Verification items for the finished model (mm, model axes). A direction names the side the tool comes from. Round coordinates to 2 decimals unless told otherwise and drop trailing zeros. Write each loop counter-clockwise with the first axis right and the second up, starting at its lowest first coordinate (ties: lowest second). Pieces come first, ordered by that corner, then holes. Notation, with made-up numbers: (-5.5, 40.25) -> (4.5, 40.25) arc R29 cw to (4.5, 70.25) -> close; hole circle Ø6 at (54, 4.25). An arc over 180 degrees is marked (long way). Answer as a JSON object with one key per item and string values. Group by question number.
(1) Scan lines: L1, parallel to Y at x = 12.5, z = 0.6; L2, parallel to Z at x = -0.75, y = -2.5; L3, parallel to Y at x = 4, z = 6. Record each from-to range of solid material in increasing order. Write a range as from..to.
(2) Draft check along Y on faces 1 (the face through (13.31, 19.25, 0.76)), 2 (the face through (-14, -7, 1)), 3 (the face through (-0.71, 16.5, 14.96)), 4 (the face through (-9, 11, 5)). Enter one of: released by +Y, released by -Y, zero draft, split by the parting line, or undercut.
(3) Set-up check for faces 5 (the face through (0, -10, 2)), 6 (the face through (-1, 15, 11.5)), 7 (the face through (0, 16.117, 5)), 8 (the face through (9, 11, 5)): record each of +Z, -Z, +X, -X, +Y, -Y from which the full face is reachable in a straight line by a thin tool's end or side.
(4) Sectioned sample at B-B on y = -6. Record the cut outline in (x, z).
(5) Sectioned sample at A-A on x = 12.5. Record the cut outline in (y, z), and give its area (3 significant figures).
(6) Sectioned sample at D-D on y = 10. Record the cut outline in (x, z).
(7) Gauge pin test, flat ends, axial feed: pin 1 Ø2.5 at (x, z) = (0.5, 5.5) entering from +Y; pin 2 Ø0.6 at (y, z) = (-10.5, 2) entering from -X; pin 3 Ø6 at (x, z) = (7, 10) entering from -Y; pin 4 Ø5.5 at (x, y) = (-1, 9) entering from -Z. Record the tip position at first contact, or that the pin passes through.
(8) Sectioned sample at C-C on z = 5.75. Record the cut outline in (x, y), and give its area (3 significant figures).
```python
from build123d import *

# Parameters (mm, degrees)
SKETCH_1_W          = 30
SKETCH_1_H          = 40
EXTRUDE_1_DEPTH     = 1.5
SKETCH_2_R          = 1.5
CUT_EXTRUDE_1_DEPTH = 2.5
SKETCH_3_W          = 18
SKETCH_3_H          = 10
EXTRUDE_2_DEPTH     = 8
SKETCH_4_R          = 5
EXTRUDE_3_DEPTH     = 2
SKETCH_5_R          = 3.78256648
EXTRUDE_4_DEPTH     = 1
SKETCH_6_R          = 5.431564172
EXTRUDE_5_DEPTH     = 5
SKETCH_7_W          = 12
SKETCH_7_H          = 12
EXTRUDE_6_DEPTH     = 0.5


with BuildPart() as part:
    # 草图1 → 凸台-拉伸1 (new body)
    with BuildSketch(Plane.XY):
        Rectangle(SKETCH_1_W, SKETCH_1_H)
    extrude(amount=EXTRUDE_1_DEPTH)

    # 草图2 → 切除-拉伸1 (cut, through all)
    with BuildSketch(Plane.XY.offset(1.5)):
        with Locations((-12.5, 17.989454292)):
            Circle(SKETCH_2_R)
        with Locations((12.5, 17.989454292)):
            Circle(SKETCH_2_R)
        with Locations((-12.5, -7.010545708)):
            Circle(SKETCH_2_R)
        with Locations((12.5, -7.010545708)):
            Circle(SKETCH_2_R)
    extrude(amount=-CUT_EXTRUDE_1_DEPTH, mode=Mode.SUBTRACT)

    # 草图3 → 凸台-拉伸2 (add)
    with BuildSketch(Plane.XY.offset(1.5)):
        with Locations((0, 11.11683457)):
            Rectangle(SKETCH_3_W, SKETCH_3_H)
    extrude(amount=EXTRUDE_2_DEPTH)

    # 草图4 → 凸台-拉伸3 (add)
    with BuildSketch(Plane.XY.offset(9.5)):
        with Locations((0, 11.11683457)):
            Circle(SKETCH_4_R)
    extrude(amount=EXTRUDE_3_DEPTH)

    # 草图5 → 凸台-拉伸4 (add)
    with BuildSketch(Plane.XY.offset(11.5)):
        with Locations((0, 11.11683457)):
            Circle(SKETCH_5_R)
    extrude(amount=EXTRUDE_4_DEPTH)

    # 草图6 → 凸台-拉伸5 (add)
    with BuildSketch(Plane.XY.offset(12.5)):
        with Locations((0, 11.11683457)):
            Circle(SKETCH_6_R)
    extrude(amount=EXTRUDE_5_DEPTH)

    # 草图7 → 凸台-拉伸6 (add)
    with BuildSketch(Plane.XY.offset(1.5)):
        with Locations((0, -9.903085883)):
            Rectangle(SKETCH_7_W, SKETCH_7_H)
    extrude(amount=EXTRUDE_6_DEPTH)


solid = part.part
```
Computed values:
{
 "1": {"L1": "-20..-8.51, -5.51..16.49, 19.49..20", "L2": "0..1.5", "L3": "6.12..16.12"},
 "2": {"face 1": "undercut", "face 2": "undercut", "face 3": "split by the parting line", "face 4": "zero draft"},
 "3": {"face 5": "+Z, +X, -X, -Y", "face 6": "none", "face 7": "+X, -X, +Y", "face 8": "+Z, +X, +Y, -Y"},
 "4": {"outline": "(-15, 0) -> (-13.61, 0) -> (-13.61, 1.5) -> (-15, 1.5) -> close; (-11.39, 0) -> (11.39, 0) -> (11.39, 1.5) -> (6, 1.5) -> (6, 2) -> (-6, 2) -> (-6, 1.5) -> (-11.39, 1.5) -> close; (13.61, 0) -> (15, 0) -> (15, 1.5) -> (13.61, 1.5) -> close"},
 "5": {"outline": "(-20, 0) -> (-8.51, 0) -> (-8.51, 1.5) -> (-20, 1.5) -> close; (-5.51, 0) -> (16.49, 0) -> (16.49, 1.5) -> (-5.51, 1.5) -> close; (19.49, 0) -> (20, 0) -> (20, 1.5) -> (19.49, 1.5) -> close", "area": "51.0 mm2"},
 "6": {"outline": "(-15, 0) -> (15, 0) -> (15, 1.5) -> (9, 1.5) -> (9, 9.5) -> (4.87, 9.5) -> (4.87, 11.5) -> (3.61, 11.5) -> (3.61, 12.5) -> (5.32, 12.5) -> (5.32, 17.5) -> (-5.32, 17.5) -> (-5.32, 12.5) -> (-3.61, 12.5) -> (-3.61, 11.5) -> (-4.87, 11.5) -> (-4.87, 9.5) -> (-9, 9.5) -> (-9, 1.5) -> (-15, 1.5) -> close"},
 "7": {"pin 1": "y = 16.12", "pin 2": "x = -6", "pin 3": "y = 6.12", "pin 4": "z = 0"},
 "8": {"outline": "(-9, 6.12) -> (9, 6.12) -> (9, 16.12) -> (-9, 16.12) -> close", "area": "180 mm2"}
}
